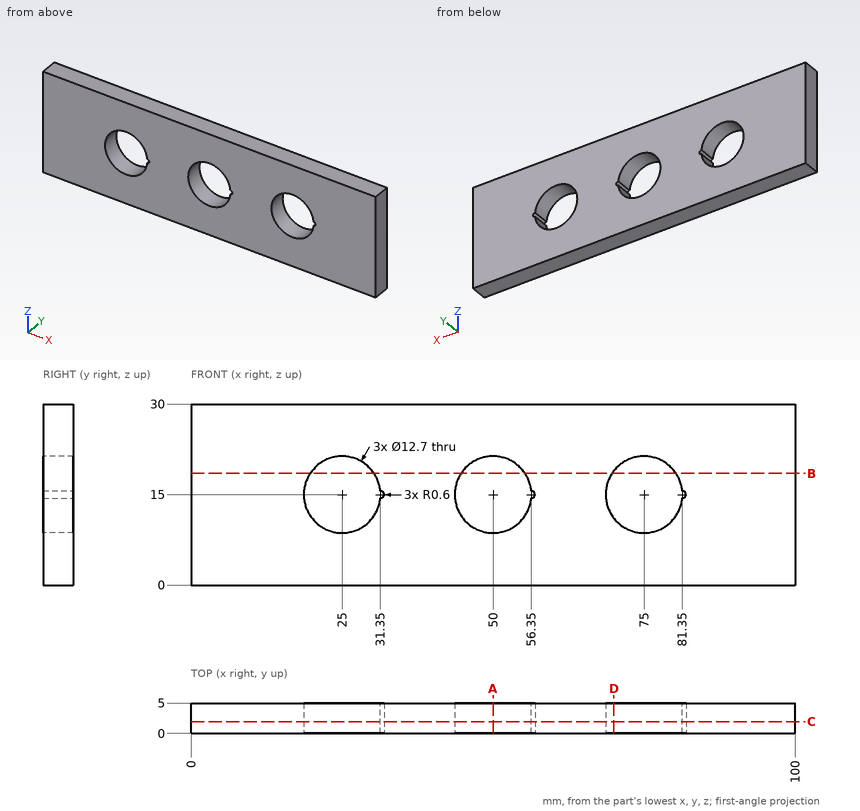
Could you check a few things on this drawing? It's one solid part, dimensions in mm from its lowest x, y, z. Coordinates: 2 decimals unless noted, no trailing zeros. Order: outer loops, then holes, each group sorted by start corner. A loop starts at its lowest first (then second) coordinate and runs counter-clockwise, first axis right, second up.
1) I need wall thicknesses on line 1 (Z direction, x = 75, y = 2.55); line 2 (X direction, y = 1.95, z = 9.5); line 3 (X direction, y = 3.4, z = 16). Which ranges of each line are inside material? Lowest first, please.
2) Will this pin go through, and if not, where does the flat tip stop? pin 1 (7.5 mm diameter, centred on x = 25, z = 15, fed in from -Y).
3) Imagine slicing it at C-C on y = 1.95. List the corners of the cut face in (x, z) for me.
4) Imagine slicing it at D-D on x = 70. List the corners of the cut face in (y, z) for me, and give its area (3 significant figures).
5) Imagine slicing it at B-B on z = 18.5. List the corners of the cut face in (x, y) for me, and give its area (3 significant figures).
6) Imagine slicing it at A-A on x = 50. List the corners of the cut face in (y, z) for me.
Response values:
1. line 1: z = 0 to 8.65, 21.35 to 30
1. line 2: x = 0 to 21.83, 28.17 to 46.83, 53.17 to 71.83, 78.17 to 100
1. line 3: x = 0 to 18.73, 31.27 to 43.73, 56.27 to 68.73, 81.27 to 100
2. pin 1: passes through
3. outline: (0, 0) - (100, 0) - (100, 30) - (0, 30) - close; hole (31.32, 14.4) arc R0.6 ccw (long way) to (31.32, 15.6) arc R6.35 ccw (long way) to start; hole (56.32, 14.4) arc R0.6 ccw (long way) to (56.32, 15.6) arc R6.35 ccw (long way) to start; hole (81.32, 14.4) arc R0.6 ccw (long way) to (81.32, 15.6) arc R6.35 ccw (long way) to start
4. outline: (0, 0) - (5, 0) - (5, 11.09) - (0, 11.09) - close; (0, 18.91) - (5, 18.91) - (5, 30) - (0, 30) - close
4. area: 111 mm2
5. outline: (0, 0) - (19.7, 0) - (19.7, 5) - (0, 5) - close; (30.3, 0) - (44.7, 0) - (44.7, 5) - (30.3, 5) - close; (55.3, 0) - (69.7, 0) - (69.7, 5) - (55.3, 5) - close; (80.3, 0) - (100, 0) - (100, 5) - (80.3, 5) - close
5. area: 341 mm2
6. outline: (0, 0) - (5, 0) - (5, 8.65) - (0, 8.65) - close; (0, 21.35) - (5, 21.35) - (5, 30) - (0, 30) - close
